from build123d import *

# Parameters (mm, degrees)
SKETCH_1_W          = 65
SKETCH_1_H          = 24
EXTRUDE_1_DEPTH     = 13
SKETCH_2_W          = 61
SKETCH_2_H          = 24
CUT_EXTRUDE_1_DEPTH = 11
SKETCH_14_R         = 2.5
CUT_EXTRUDE_2_DEPTH = 2


with BuildPart() as part:
    # 草圖1 → 填料-伸長1 (new body)
    with BuildSketch(Plane.XY):
        with Locations((-32.5, 12)):
            Rectangle(SKETCH_1_W, SKETCH_1_H)
    extrude(amount=EXTRUDE_1_DEPTH)

    # 草圖2 → 除料-伸長1 (cut)
    with BuildSketch(Plane.XY.offset(13)):
        with Locations((-32.5, 12)):
            Rectangle(SKETCH_2_W, SKETCH_2_H)
    extrude(amount=-CUT_EXTRUDE_1_DEPTH, mode=Mode.SUBTRACT)

    # 草圖14 → 除料-伸長2 (cut)
    with BuildSketch(Plane(origin=(0, 0, 0), x_dir=(-1, 0, 0), z_dir=(0, 0, -1))):
        with Locations((10, 19)):
            Circle(SKETCH_14_R)
        with Locations((20, 5)):
            Circle(SKETCH_14_R)
    extrude(amount=-CUT_EXTRUDE_2_DEPTH, mode=Mode.SUBTRACT)


solid = part.part
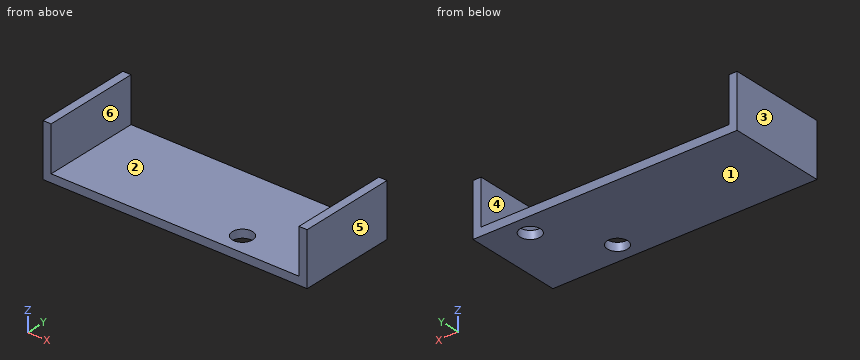
Verification items for the finished model (mm, model axes). Face numbers are marked on the shaded views. A direction names the side the tool comes from. Coordinates: 2 decimals unless noted, no trailing zeros. Loops run counter-clockwise (first coordinate to the right, second up) from the corner with the lowest first, then second, coordinate; pieces in that order, holes last. Notation, with made-up numbers: M 84,35.5 L 102,35.5 A16 ccw 102,51.5 Z; hole C -18,84 d9. An arc over 180 degrees is marked long. One line per item, written item: value.
1. Section check C-C on z = 9. Record the cut outline in (x, y).
Answers follow:
outline: M -65,0 L -63,0 L -63,24 L -65,24 Z; M -2,0 L 0,0 L 0,24 L -2,24 Z
2. Gauge pin test, flat ends, axial feed: P1, Ø5, axis at x = -19, z = 2.5, coming from the -Y side; P2, Ø8, axis at x = -27.5, y = 19, coming from the +Z side; P3, Ø4.5, axis at x = -20, y = 5, coming from the -Z side. Record the tip position at first contact, or that the pin passes through.
Answers follow:
P1: y = 0
P2: z = 2
P3: through
3. Section check A-A on y = 5. Record the cut outline in (x, z).
Answers follow:
outline: M -65,0 L -22.5,0 L -22.5,2 L -63,2 L -63,13 L -65,13 Z; M -17.5,0 L 0,0 L 0,13 L -2,13 L -2,2 L -17.5,2 Z
4. Section check B-B on x = -10. Record the cut outline in (y, z).
Answers follow:
outline: M 0,0 L 16.5,0 L 16.5,2 L 0,2 Z; M 21.5,0 L 24,0 L 24,2 L 21.5,2 Z
5. Material ranges on line 1 along Y through (x, z) = (-10, 1.2); line 2 along X through (y, z) = (8.75, 4.25); line 3 along Y through (x, z) = (-20, 0.6), recorded low to high. Write a range as from..to.
Answers follow:
line 1: 0..16.5, 21.5..24
line 2: -65..-63, -2..0
line 3: 0..2.5, 7.5..24
6. Mould release check, pull along X, two halves, no side actions. Record for the marked faces 1, 2, 3 and 4: pulls with the +X half, pulls with the -X half, needs draft (parallel to the pull), parting line crosses it, or undercut.
Answers follow:
face 1: needs draft
face 2: undercut
face 3: pulls with the -X half
face 4: undercut
7. Section check D-D on y = 10. Record the cut outline in (x, z).
Answers follow:
outline: M -65,0 L 0,0 L 0,13 L -2,13 L -2,2 L -63,2 L -63,13 L -65,13 Z
8. Set-up check for the marked faces 5 and 6: record each of +Z, -Z, +X, -X, +Y, -Y from which the full face is reachable in a straight line by a thin tool's end or side.
Answers follow:
face 5: +Z, -Z, +X, +Y, -Y
face 6: +Z, +Y, -Y
